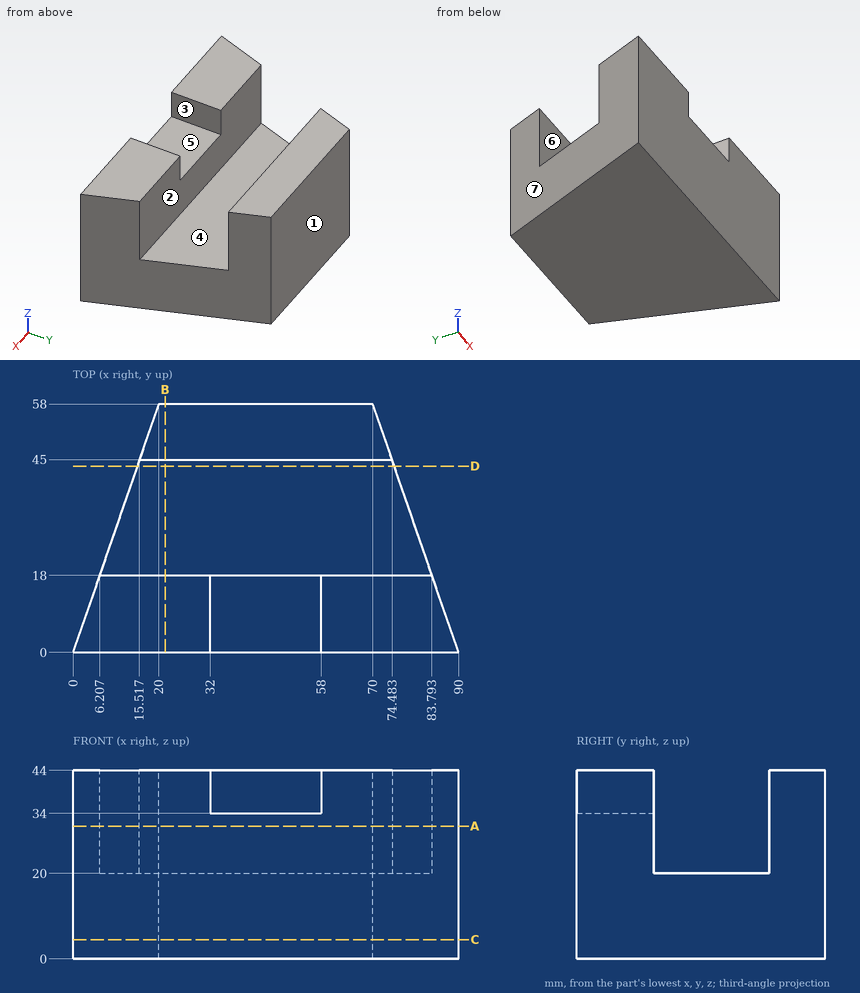
Can you work these out from the drawing? Everything is in mm from the part's minimum corner. A direction names the side the tool comes from. Round coordinates to 2 decimals unless told otherwise and drop trailing zeros. Order: outer loops, then holes, each group sorted by start corner. A loop starts at its lowest first (then second) coordinate and runs counter-clockwise, first axis right, second up. Notation, with made-up numbers: M 46,41 L 66,41 A30 cw 66,72 Z; hole C 78,82 d5. An arc over 180 degrees is marked long. Answer as CSV lines item,"result".
Item 1: Imagine slicing it at A-A on z = 31. List the corners of the cut face in (x, y) for me.
From the geometry:
outline,"M 0,0 L 90,0 L 83.79,18 L 6.21,18 Z; M 15.52,45 L 74.48,45 L 70,58 L 20,58 Z"
Item 2: Which directions (+Z, -Z, +X, -X, +Y, -Y) give clear straight access to the entire face, cutting with the end or side of a thin tool? Please do the marked faces 5, 6 and 7.
From the geometry:
face 5,"+Z, -Y"
face 6,"+Z, +X, -X"
face 7,"+Z, -Z, -X, +Y"
Item 3: Imagine slicing it at C-C on z = 4.5. List the corners of the cut face in (x, y) for me, and give its area (3 significant figures).
From the geometry:
outline,"M 0,0 L 90,0 L 70,58 L 20,58 Z"
area,"4,060 mm2"
Item 4: We'd pull the mould along Y, two halves only. Please class the marked faces 1, 2, 3 and 4: +Y half, -Y half, draft (parallel to the pull), parting line (faces both ways), or undercut.
From the geometry:
face 1,"+Y half"
face 2,"undercut"
face 3,"draft"
face 4,"undercut"
Item 5: For pin 1 (5 mm diameter, centred on y = 7, z = 36.5, fed in from +X); pin 2 (12 mm diameter, centred on x = 61, y = 29.5, fed in from +Z); pin 3 (1 mm diameter, centred on y = 18, z = 21, fed in from -X) (1 decimal), each with a flat end and sliding along its axis, tell me the tip position at first contact or that it passes through.
From the geometry:
pin 1,"x = 88.45"
pin 2,"z = 20"
pin 3,"x = 6"
Item 6: Imagine slicing it at B-B on x = 21.5. List the corners of the cut face in (y, z) for me, and give its area (3 significant figures).
From the geometry:
outline,"M 0,0 L 58,0 L 58,44 L 45,44 L 45,20 L 18,20 L 18,44 L 0,44 Z"
area,"1,900 mm2"
Item 7: Please list where these lines run through material, in increasing order: L1, parallel to Y at x = 46.5, z = 20.5; L2, parallel to Z at x = 77, y = 25; L3, parallel to Y at x = 80.5, z = 33.5. Write a range as [from, to].
From the geometry:
L1,"[0, 18], [45, 58]"
L2,"[0, 20]"
L3,"[0, 18]"
Item 8: Imagine slicing it at D-D on y = 43.5. List the corners of the cut face in (x, z) for me.
From the geometry:
outline,"M 15,0 L 75,0 L 75,20 L 15,20 Z"
